Model file for the job. Use its own axes, mm. Face numbers are marked on the shaded views. A direction names the side the tool comes from. Round coordinates to 2 decimals unless told otherwise and drop trailing zeros. Order: outer loops, then holes, each group sorted by start corner. A loop starts at its lowest first (then second) coordinate and runs counter-clockwise, first axis right, second up. Notation, with made-up numbers: M 0.5,87.25 L 8.5,87.25 A23 cw 8.5,125.25 Z; hole C 6,60 d7. An arc over 180 degrees is marked long. Return JSON: item names as keys, results as strings. Group by question number.
Item 1: Pin check, flat tips, straight feed: pin 1 Ø2.5 at (x, y) = (-0.5, -3) entering from -Z; pin 2 Ø7.5 at (x, y) = (-4.5, -3.5) entering from +Z (3 decimals); pin 3 Ø4 at (x, y) = (10, -10.5) entering from -Z. Stop position of each tip, or through.
Item 2: Slice it at D-D on z = 54.5. Write the cut outline in (x, y), then the cut area to 3 significant figures.
Item 3: Probe line 1 along X through (y, z) = (2, 0); line 2 along Z through (x, y) = (0, -2.95) (3 decimals); line 3 along Z through (x, y) = (0, 6) (3 decimals). List the from-to ranges inside material, lowest first.
Item 4: Pull direction X, two halves, no side cores. Call the marked faces 3, 4, 5 and 6: pulls with the +X half, pulls with the -X half, needs draft (parallel to the pull), parting line crosses it, or undercut.
Item 5: Slice it at C-C on y = 1.25. Write the cut outline in (x, z) (3 decimals), then the cut area to 3 significant figures.
Item 6: Which spindle directions (+Z, -Z, +X, -X, +Y, -Y) get a long thin tool onto all of the face, cutting with end or side? Do the marked faces 1 and 2. Say none if no direction does.
Item 7: Slice it at A-A on x = 17. Give the number of separate pieces and of enclosed holes in the cut face, then the cut area to 3 significant figures.
from build123d import *

# Parameters (mm, degrees)
F0_R          = 37.5
F0_R_2        = 25
F1_DEPTH      = 5
F2_W          = 5
F2_H          = 10
F3_DEPTH      = 5
F4_R          = 2.49999
F5_R          = 37.5
F5_R_2        = 25
F6_DEPTH      = 10
F6_DEPTH_BACK = 15
F7_W          = 50
F7_H          = 40
F8_DEPTH      = 15
F8_DEPTH_BACK = 10
F9_W          = 25
F9_H          = 30
F10_DEPTH     = 25
F11_R         = 12.49999
F12_R         = 5
F13_DEPTH     = 62.501


# Not quite as in the source:
# - a fillet or chamfer is up to 0.001 mm smaller than in the source, because OpenCascade refuses the exact size


with BuildPart() as f1:
    # F0 (on Front) → F1 (new body)
    with BuildSketch(Plane.XZ):
        Circle(F0_R)
        Circle(F0_R_2, mode=Mode.SUBTRACT)
    extrude(amount=F1_DEPTH)

    # F2 (on Front) → F3 (join)
    with BuildSketch(Plane.XZ):
        with Locations((0, 25)):
            Rectangle(F2_W, F2_H)
    extrude(amount=F3_DEPTH)

    # F4 (radius 2.5 in the source; OpenCascade refuses exactly that, so slightly less here)
    f4_edges = [f1.edges().sort_by_distance(p)[0] for p in [
        (-2.5, -5, 22.437343),
        (2.5, -5, 22.437343),
        (-2.5, 0, 22.437343),
        (2.5, 0, 22.437343),
    ]]
    fillet(f4_edges, radius=F4_R)

    # F5 (on face) → F6 (join, two sides)
    with BuildSketch(Plane.XZ.offset(5)) as f6_sk:
        Circle(F5_R)
        Circle(F5_R_2, mode=Mode.SUBTRACT)
    extrude(amount=F6_DEPTH)
    extrude(f6_sk.sketch, amount=-F6_DEPTH_BACK)

    # F7 (on Front) → F8 (join, two sides)
    with BuildSketch(Plane.XZ) as f8_sk:
        with Locations((0, 45.1250001788)):
            Rectangle(F7_W, F7_H)
    extrude(amount=F8_DEPTH)
    extrude(f8_sk.sketch, amount=-F8_DEPTH_BACK)

    # F9 (on face) → F10 (cut)
    with BuildSketch(Plane.XZ.offset(15)):
        with Locations((0, 50.1250001788)):
            Rectangle(F9_W, F9_H)
    extrude(amount=-F10_DEPTH, mode=Mode.SUBTRACT)

    # F11 (radius 12.5 in the source; OpenCascade refuses exactly that, so slightly less here)
    f11_edges = [f1.edges().sort_by_distance(p)[0] for p in [
        (-18.75, 10, 65.125),
        (-18.75, -15, 65.125),
        (18.75, -15, 65.125),
        (18.75, 10, 65.125),
    ]]
    fillet(f11_edges, radius=F11_R)

    # F12 (on face) → F13 (cut, through all)
    with BuildSketch(Plane(origin=(-25, 0, 0), x_dir=(0, -1, 0), z_dir=(-1, 0, 0))):
        with Locations((2.5, 52.6250001788)):
            Circle(F12_R)
    extrude(amount=-F13_DEPTH, mode=Mode.SUBTRACT)


solid = f1.part
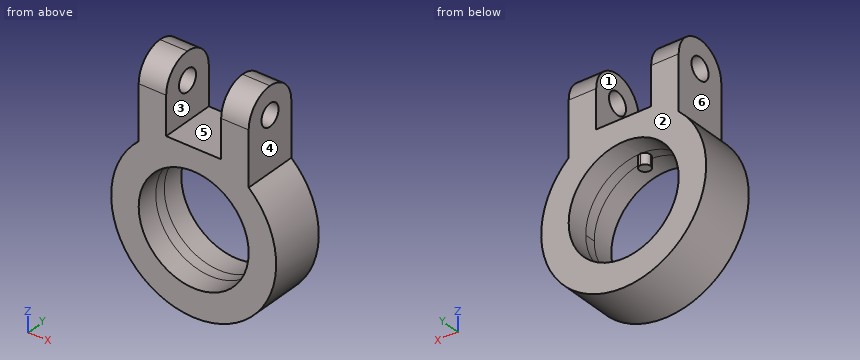
Output values:
{
 "1": {"pin 1": "z = -37.5", "pin 2": "z = 35.125", "pin 3": "z = -36.64"},
 "2": {"outline": "M -25,-14.86 L -12.5,-14.86 L -12.5,-7.14 L -25,-7.14 Z; M -25,2.14 L -12.5,2.14 L -12.5,9.86 L -25,9.86 Z; M 12.5,-14.86 L 25,-14.86 L 25,-7.14 L 12.5,-7.14 Z; M 12.5,2.14 L 25,2.14 L 25,9.86 L 12.5,9.86 Z", "area": "386 mm²"},
 "3": {"line 1": "-37.5 to -25, 25 to 37.5", "line 2": "-37.5 to -25, 20 to 35.125", "line 3": "-37.5 to -25, 25 to 35.125"},
 "4": {"face 3": "undercut", "face 4": "pulls with the +X half", "face 5": "undercut", "face 6": "pulls with the -X half"},
 "5": {"outline": "M -25,27.951 A37.5 ccw long 25,27.951 L 25,49.318 L 12.5,49.318 L 12.5,35.125 L -12.5,35.125 L -12.5,49.318 L -25,49.318 Z; M -25,55.932 L -12.5,55.932 L -12.5,64.549 L -25,64.549 Z; M 12.5,55.932 L 25,55.932 L 25,64.549 L 12.5,64.549 Z; hole C 0,0 d50", "area": "3,060 mm²"},
 "6": {"face 1": "+Z, +Y, -Y", "face 2": "+Z, -Z, +X, -X, +Y"},
 "7": {"separate pieces": "2", "enclosed holes": "1", "area": "1,400 mm²"}
}
